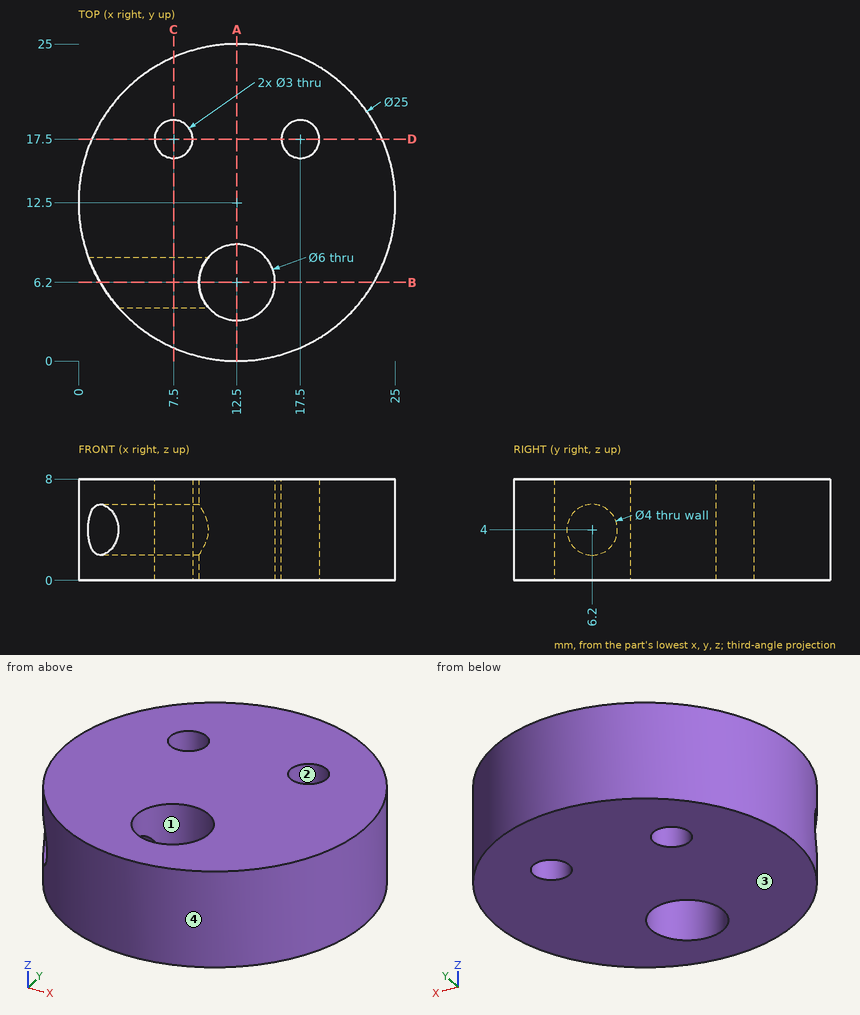
For this review, use the dimensioned drawing (mm, ordinates from the lowest corner) and the shaded views. Round coordinates to 2 decimals unless told otherwise and drop trailing zeros. Order: outer loops, then holes, each group sorted by start corner. A loop starts at its lowest first (then second) coordinate and runs counter-clockwise, first axis right, second up. Notation, with made-up numbers: M 65,8 L 80,8 A18 cw 80,14 Z; hole C -38,55.5 d9. An arc over 180 degrees is marked long. Write each question's results on one line, items separated by ' | '. Start each with the question number.
1. Add section D-D (y = 17.5). State the section outline as (x, z) points.
2. Add section A-A (x = 12.5). State the section outline as (y, z) points, then the cut area to 3 significant figures.
3. Add section C-C (x = 7.5). State the section outline as (y, z) points.
4. Add section B-B (y = 6.2). State the section outline as (x, z) points.
5. Clearance check with flat-ended pins moving along their axes: pin 1 Ø3.5 at (x, y) = (17.5, 17.5) entering from -Z; pin 2 Ø3 at (y, z) = (6, 1) entering from +X; pin 3 Ø1.5 at (x, z) = (16, 6) entering from -Y; pin 4 Ø2 at (y, z) = (19.5, 6.5) entering from -X. State where each tip first meets the part, or that it passes through.
6. Draft analysis for pull direction Y (two halves, no side actions). For the marked faces 1, 2, 3 and 4, state which applies: pulls with the +Y half, pulls with the -Y half, needs draft (parallel to the pull), parting line crosses it, or undercut.
7. To check wall thickness, follow L1, parallel to X at y = 18.5, z = 3.75; L2, parallel to X at y = 8, z = 2; L3, parallel to X at y = 16.75, z = 6. State the ranges of each line that lie inside material, in increasing order. Write a range as [from, to].
Output values:
1) outline: M 1.04,0 L 6,0 L 6,8 L 1.04,8 Z; M 9,0 L 16,0 L 16,8 L 9,8 Z; M 19,0 L 23.96,0 L 23.96,8 L 19,8 Z
2) outline: M 0,0 L 3.2,0 L 3.2,8 L 0,8 Z; M 9.2,0 L 25,0 L 25,8 L 9.2,8 Z | area: 152 mm^2
3) outline: M 1.04,0 L 16,0 L 16,8 L 1.04,8 Z; M 19,0 L 23.96,0 L 23.96,8 L 19,8 Z; hole C 6.2,4 d4
4) outline: M 1.7,0 L 9.5,0 L 9.5,2 L 1.7,2 Z; M 1.7,6 L 9.5,6 L 9.5,8 L 1.7,8 Z; M 15.5,0 L 23.3,0 L 23.3,8 L 15.5,8 Z
5) pin 1: z = 0 | pin 2: x = 23.96 | pin 3: y = 0.31 | pin 4: x = 1.53
6) face 1: undercut | face 2: undercut | face 3: needs draft | face 4: parting line crosses it
7) L1: [1.53, 6.38], [8.62, 16.38], [18.62, 23.47] | L2: [0.84, 10.1], [14.9, 24.16] | L3: [0.74, 6.2], [8.8, 16.2], [18.8, 24.26]
